Autodesk Inventor part; units mm, degrees
ref_plane "YZ Plane" through (0, 0, 0) normal (1, 0, 0) x (0, 1, 0)
ref_plane "XZ Plane" through (0, 0, 0) normal (0, 1, 0) x (-1, 0, 0)
ref_plane "XY Plane" through (0, 0, 0) normal (0, 0, 1) x (1, 0, 0)
sketch "Эскиз1" plane through (0, 0, 0) normal (0, 1, 0) x (-1, 0, 0)
  line L0 (30, 181.2) -> (30, 186.2)
  line L1 (30, 186.2) -> (95, 186.2)
  line L2 (95, 186.2) -> (95, 90.2)
  line L3 (95, 90.2) -> (30, 90.2)
  line L4 (30, 90.2) -> (30, 95.2)
  line L5 (30, 95.2) -> (90, 95.2)
  line L6 (90, 95.2) -> (90, 181.2)
  line L7 (90, 181.2) -> (30, 181.2)
  line L8 (0, -115.5707) -> (0, 259.8393)
  line L9 (70, 181.2) -> (-70, 181.2)
  point P0 (0, 0)
  dimension "d0" = 5
  dimension "d1" = 5
  dimension "d2" = 5
  dimension "d3" = 86
  dimension "d4" = 180
  dimension "d5" = 60
revolve "Вращение1" add sketch "Эскиз1" angle 360 about axis through (0, 0, -115.5707) along (0, 0, 1)
sketch "Эскиз2" plane through (0, 0, 186.2) normal (0, 0, 1) x (1, 0, 0)
  line L0 (-15, 72.7645) -> (-15, 82.7645)
  line L1 (15, 82.7645) -> (-15, 82.7645)
  line L2 (15, 72.7645) -> (15, 82.7645)
  line L3 (-15, 72.7645) -> (15, 72.7645)
  line L4 (-15.5, 83.2645) -> (-15.5, 72.2645)
  line L5 (-15.5, 72.2645) -> (15.5, 72.2645)
  line L6 (15.5, 72.2645) -> (15.5, 83.2645)
  line L7 (15.5, 83.2645) -> (-15.5, 83.2645)
  point P0 (0, 0)
  dimension "d7" = 0.5
extrude "Выдавливание1" cut sketch "Эскиз2" against normal blind 7 contours L0 L1 L2 L3 | L7 L6 L5 L4
sketch "Эскиз3" plane through (0, 0, 90.2) normal (0, 0, -1) x (-1, 0, 0)
  line L0 (15, 82.7645) -> (-15, 82.7645)
  line L1 (-15, 72.7645) -> (15, 72.7645)
  line L2 (15, 72.7645) -> (15, 82.7645)
  line L3 (-15, 72.7645) -> (-15, 82.7645)
  point P0 (0, 0)
extrude "Выдавливание2" add sketch "Эскиз3" along normal blind 130
sketch "Эскиз4" plane through (-15, 82.7645, 90.2) normal (0, 1, 0) x (1, 0, 0)
  line L0 (30, 0) -> (30, 130)
  line L1 (0, 0) -> (0, 130)
  arc A0 (30, 115) -> (0, 115) centre (15, 115) ccw
  line L2 (30, 130) -> (0, 130)
  circle A1 centre (15, 115) radius 10
  point P0 (15, 90.2)
  point P1 (15, 130)
  dimension "d15" = 20
extrude "Выдавливание3" cut sketch "Эскиз4" against normal blind 24.5
ref_plane "РабПлоскость1" through (0, 0, 138.2) normal (0, 0, -1) x (-1, 0, 0)
sketch "Эскиз5" plane through (0, 0, 138.2) normal (0, 0, -1) x (-1, 0, 0)
  line L0 (0, 0) -> (-41.3014, 113.4746)
  line L1 (-41.3014, 113.4746) -> (-113.4746, 41.3014)
  line L2 (-113.4746, 41.3014) -> (0, 0)
  line L3 (0, 0) -> (-77.388, 77.388) construction
  line L4 (0, 0) -> (-129.096, 0) construction
  dimension "d18" = 50
  dimension "d19" = 45
extrude "Выдавливание4" cut sketch "Эскиз5" along normal up to surface (43 mm away)
sketch "Эскиз6" plane through (0, 0, 138.2) normal (0, 0, -1) x (-1, 0, 0)
  arc A0 (-30.7818, 84.5723) -> (-84.5723, 30.7818) centre (0, 0) ccw
  line L0 (-30.7818, 84.5723) -> (-32.4919, 89.2708)
  arc A1 (-32.4919, 89.2708) -> (-89.2708, 32.4919) centre (0, 0) ccw
  line L1 (-89.2708, 32.4919) -> (-84.5723, 30.7818)
extrude "Выдавливание5" cut sketch "Эскиз6" against normal up to surface (43 mm away)
pattern_circular "Круговой массив1" count 4 over 360 about axis through (0, 0, 138.2) along (0, 0, -1) of "Выдавливание4", "Выдавливание5"
properties part number "outer_part"
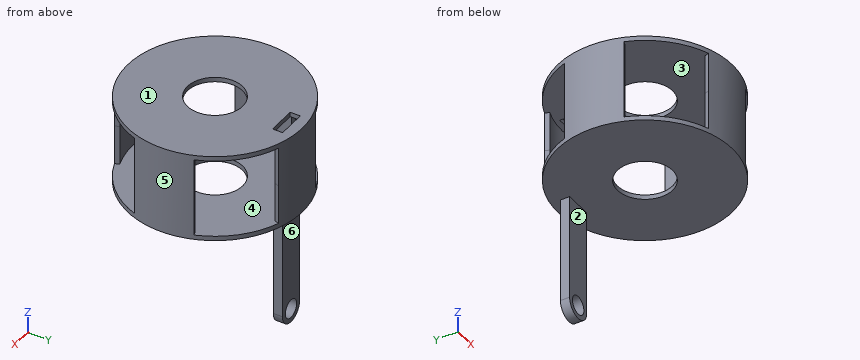
Design review of the part built by this model. Coordinates are the model's own, in mm. Face numbers are marked on the shaded views. A direction names the side the tool comes from. Coordinates: 2 decimals unless noted, no trailing zeros. Loops run counter-clockwise (first coordinate to the right, second up) from the corner with the lowest first, then second, coordinate; pieces in that order, holes last. Notation, with made-up numbers: (-33, -28.75) -> (26, -28.75) arc R25 ccw to (26, 10.25) -> close; hole circle Ø11 at (-37, 2). An arc over 180 degrees is marked (long way). Answer as a JSON object with one key per item and string values.
Q1. Tool access review of the marked faces 4, 5 and 6: name each direction out of +Z, -Z, +X, -X, +Y, -Y from which nothing blocks a thin tool from reaching the whole face with its end or side.
Answer block:
{"face 4": "none", "face 5": "+Z, -Z", "face 6": "-Z, +X, -X, +Y"}
Q2. Clearance check with flat-ended pins moving along their axes: pin 1 Ø5 at (y, z) = (78, 38) entering from -X; pin 2 Ø5 at (x, y) = (-23, -13) entering from -Z; pin 3 Ø24 at (x, z) = (7, 15.5) entering from +Y; pin 4 Ø24 at (x, z) = (-4.5, 18.5) entering from -Y. State where each tip first meets the part, or that it passes through.
Answer block:
{"pin 1": "stops at x = -15", "pin 2": "passes through", "pin 3": "stops at y = 82.76", "pin 4": "stops at y = 72.76"}
Q3. Take a section at C-C on y = 78. Give the boundary of the cut face in (x, z), plus the area to 3 significant figures.
Answer block:
{"outline": "(-54.23, 90.2) -> (-15, 90.2) -> (-15, -24.8) arc R15 ccw to (15, -24.8) -> (15, 90.2) -> (54.23, 90.2) -> (54.23, 95.2) -> (-54.23, 95.2) -> close; (-54.23, 181.2) -> (-15.5, 181.2) -> (-15.5, 186.2) -> (-54.23, 186.2) -> close; (15.5, 181.2) -> (54.23, 181.2) -> (54.23, 186.2) -> (15.5, 186.2) -> close; hole circle Ø20 at (0, -24.8)", "area": "4,420 mm^2"}
Q4. The part is to be moulded in two halves that separate along Z. For the marked faces 1, 2 and 3, say which applies: +Z half, -Z half, draft (parallel to the pull), parting line (faces both ways), or undercut.
Answer block:
{"face 1": "+Z half", "face 2": "draft", "face 3": "undercut"}
Q5. Take a section at A-A on x = 0. Give the boundary of the cut face in (y, z), plus the area to 4 significant figures.
Answer block:
{"outline": "(-95, 90.2) -> (-30, 90.2) -> (-30, 95.2) -> (-90, 95.2) -> (-90, 181.2) -> (-30, 181.2) -> (-30, 186.2) -> (-95, 186.2) -> close; (30, 90.2) -> (72.76, 90.2) -> (72.76, -14.8) -> (82.76, -14.8) -> (82.76, 90.2) -> (95, 90.2) -> (95, 186.2) -> (83.26, 186.2) -> (83.26, 181.2) -> (90, 181.2) -> (90, 95.2) -> (30, 95.2) -> close; (30, 181.2) -> (72.26, 181.2) -> (72.26, 186.2) -> (30, 186.2) -> close; (72.76, -39.8) -> (82.76, -39.8) -> (82.76, -34.8) -> (72.76, -34.8) -> close", "area": "3,205 mm^2"}
Q6. Take a section at D-D on z = 144. Give the boundary of the cut face in (x, y).
Answer block:
{"outline": "(-89.27, -32.49) -> (-84.57, -30.78) arc R90 cw to (-84.57, 30.78) -> (-89.27, 32.49) arc R95 ccw to start; (-32.49, -89.27) arc R95 ccw to (32.49, -89.27) -> (30.78, -84.57) arc R90 cw to (-30.78, -84.57) -> close; (-32.49, 89.27) -> (-30.78, 84.57) arc R90 cw to (30.78, 84.57) -> (32.49, 89.27) arc R95 ccw to start; (84.57, -30.78) -> (89.27, -32.49) arc R95 ccw to (89.27, 32.49) -> (84.57, 30.78) arc R90 cw to start"}
Q7. To check wall thickness, follow L1, parallel to Y at x = 0, z = 183; L2, parallel to Z at x = -37.5, y = 1; L3, parallel to Y at x = 3, z = 117. State the ranges of each line that lie inside material, in increasing order.
Answer block:
{"L1": "y = -95 to -30, 30 to 72.26, 83.26 to 95", "L2": "z = 90.2 to 95.2, 181.2 to 186.2", "L3": "y = -94.95 to -89.95, 89.95 to 94.95"}
Q8. Take a section at B-B on y = 0. Give the boundary of the cut face in (x, z).
Answer block:
{"outline": "(-95, 90.2) -> (-30, 90.2) -> (-30, 95.2) -> (-90, 95.2) -> (-90, 181.2) -> (-30, 181.2) -> (-30, 186.2) -> (-95, 186.2) -> close; (30, 90.2) -> (95, 90.2) -> (95, 186.2) -> (30, 186.2) -> (30, 181.2) -> (90, 181.2) -> (90, 95.2) -> (30, 95.2) -> close"}
